Verification items for the finished model (mm, model axes). Face numbers are marked on the shaded views. Give positions to 0.01 mm unless a question says otherwise; leave off trailing zeros. Write each loop counter-clockwise with the first axis right and the second up, starting at its lowest first coordinate (ties: lowest second). Pieces come first, ordered by that corner, then holes. Notation, with made-up numbers: (29.5, 30.5) -> (68.5, 30.5) arc R12 cw to (68.5, 35.5) -> close; hole circle Ø4 at (42, 7). An arc over 180 degrees is marked (long way). Use one line per item in the form item = value. Start each with the question number.
(1) Section check B-B, the plane z = 2. Record the cut outline in (x, y).
(2) Scan lines: L1, parallel to Y at x = 0, z = 16.5; L2, parallel to X at y = 0, z = 22.25; L3, parallel to X at y = 0, z = 13.75. Record each from-to range of solid material in increasing order.
(3) Release check for a two-part mould opening along Z. For the marked faces 1, 2, 3 and 4 record: pulls with the +Z half, pulls with the -Z half, needs draft (parallel to the pull), parting line crosses it, or undercut.
(4) Depth check by flat-ended pin: pin 1 Ø8 at (x, z) = (-6.5, 12) entering from +Y; pin 2 Ø6 at (y, z) = (-1.5, 4.5) entering from -X; pin 3 Ø2 at (y, z) = (0.5, 19.5) entering from -X; pin 4 Ø1.8 at (x, y) = (0, 0) entering from +Z. Enter the tip coordinate at first touch or a pass-through.
(5) Section check A-A, the plane z = 15.75. Record the cut outline in (x, y).
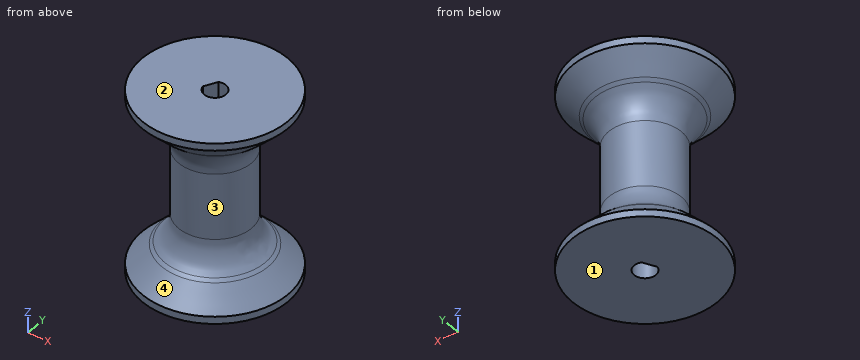
from build123d import *

# Parameters (mm, degrees)
SKETCH1_R           = 10
BOSS_EXTRUDE1_DEPTH = 5
SKETCH3_R           = 5
BOSS_EXTRUDE3_DEPTH = 15
SKETCH4_R           = 10
BOSS_EXTRUDE4_DEPTH = 5
CUT_EXTRUDE1_DEPTH  = 26
CHAMFER3_SIZE       = 4
FILLET6_R           = 5
FILLET7_R           = 5


with BuildPart() as part:
    # Sketch1 → Boss-Extrude1 (new body)
    with BuildSketch(Plane.XY):
        Circle(SKETCH1_R)
    extrude(amount=BOSS_EXTRUDE1_DEPTH)

    # Sketch3 → Boss-Extrude3 (add)
    with BuildSketch(Plane.XY.offset(5)):
        Circle(SKETCH3_R)
    extrude(amount=BOSS_EXTRUDE3_DEPTH)

    # Sketch4 → Boss-Extrude4 (add)
    with BuildSketch(Plane.XY.offset(20)):
        Circle(SKETCH4_R)
    extrude(amount=BOSS_EXTRUDE4_DEPTH)

    # Sketch5 → Cut-Extrude1 (cut)
    with BuildSketch(Plane(origin=(0, 0, 0), x_dir=(-1, 0, 0), z_dir=(0, 0, -1))):
        with BuildLine():
            Line((0.567187137, 1.388631971), (1.468830879, -0.304197058))
            ThreePointArc((1.468830879, -0.304197058), (-1.323918378, -0.705152558), (0.567187137, 1.388631971))
        make_face()
    extrude(amount=-CUT_EXTRUDE1_DEPTH, mode=Mode.SUBTRACT)

    # Chamfer3
    chamfer3_edges = [part.edges().sort_by_distance(p)[0] for p in [
        (-10, 0, 20),
        (-10, 0, 5),
    ]]
    chamfer(chamfer3_edges, length=CHAMFER3_SIZE)

    # Fillet6
    # the kernel refuses this fillet: 5 mm, written as the material it takes off along each edge
    with BuildSketch(Plane(origin=(0, 0, 20), x_dir=(1, 0, 0), z_dir=(0, -1, 0))) as fillet6_piece_1:
        with BuildLine():
            CenterArc((3.777070272, 4.848138084), FILLET6_R, 284.157365729, 30.842634271)
            Line((5, 0), (5.024458595, -0.096962762))
            ThreePointArc((5.024458595, -0.096962762), (5.5, -0.1), (6, -0.1))
            Line((6, -0.1), (6.070710678, -0.070710678))
            Line((6.070710678, -0.070710678), (7.383314856, 1.2418935))
            Line((7.383314856, 1.2418935), (7.312604178, 1.312604178))
        make_face()
    revolve(axis=Axis((0, 0, 20), (0, 0, 1)), mode=Mode.SUBTRACT)
    with BuildSketch(Plane(origin=(0, 0, 5), x_dir=(1, 0, 0), z_dir=(0, -1, 0))) as fillet6_piece_2:
        with BuildLine():
            CenterArc((3.777070272, -4.848138084), FILLET6_R, 45, 30.842634271)
            Line((7.312604178, -1.312604178), (7.383314856, -1.2418935))
            Line((7.383314856, -1.2418935), (6.070710678, 0.070710678))
            Line((6.070710678, 0.070710678), (6, 0.1))
            ThreePointArc((6, 0.1), (5.5, 0.1), (5.024458595, 0.096962762))
            Line((5.024458595, 0.096962762), (5, 0))
        make_face()
    revolve(axis=Axis((0, 0, 5), (0, 0, 1)), mode=Mode.SUBTRACT)

    # Fillet7
    fillet7_edges = [part.edges().sort_by_distance(p)[0] for p in [
        (-5, 0, 5),
        (-5, 0, 20),
    ]]
    fillet(fillet7_edges, radius=FILLET7_R)


solid = part.part
Completed:
q1.outline = circle Ø18 at (0, 0); hole (-1.47, -0.3) arc R1.5 ccw (long way) to (-0.57, 1.39) -> close
q2.L1 = -5 to -1.5, 1.5 to 5
q2.L2 = -8.25 to -1.31, 1.5 to 8.25
q2.L3 = -5 to -1.31, 1.5 to 5
q3.face_1 = pulls with the -Z half
q3.face_2 = pulls with the +Z half
q3.face_3 = undercut
q3.face_4 = undercut
q4.pin_1 = 4.33
q4.pin_2 = -9.41
q4.pin_3 = -6.39
q4.pin_4 = through
q5.outline = circle Ø10 at (0, 0); hole (-1.47, -0.3) arc R1.5 ccw (long way) to (-0.57, 1.39) -> close
